from build123d import *

# Parameters (mm, degrees)
BOSS_EXTRUDE1_DEPTH = 18
SKETCH2_W           = 200
SKETCH2_H           = 118
CUT_EXTRUDE1_DEPTH  = 19
CUT_EXTRUDE2_DEPTH  = 10
SKETCH4_W           = 17.5
SKETCH4_H           = 40
SKETCH4_W_2         = 40
SKETCH4_H_2         = 17.5
SKETCH4_H_3         = 20
CUT_EXTRUDE3_DEPTH  = 19


with BuildPart() as part:
    # Sketch1 → Boss-Extrude1 (new body)
    with BuildSketch(Plane.XY):
        with BuildLine():
            Line((0, 0), (51.303021499, -140.953893118))
            Line((51.303021499, -140.953893118), (-5.078535748, -161.475101717))
            ThreePointArc((-5.078535748, -161.475101717), (-63.089907624, -263.513472234), (-48.666413819, -380))
            Line((-48.666413819, -380), (-491.60308739, -380))
            ThreePointArc((-491.60308739, -380), (-536.64849181, -170.176041514), (-749.936822659, -193.909350133))
            ThreePointArc((-749.936822659, -193.909350133), (-806.401902791, -197.329105332), (-809.82165799, -140.864025199))
            ThreePointArc((-809.82165799, -140.864025199), (-704.170284695, -71.694204299), (-578.030994047, -65.731305902))
            ThreePointArc((-578.030994047, -65.731305902), (-333.746195792, -84.570747443), (-93.969262079, -34.202014333))
            Line((-93.969262079, -34.202014333), (0, 0))
        make_face()
    extrude(amount=BOSS_EXTRUDE1_DEPTH)

    # Sketch2 → Cut-Extrude1 (cut, through all)
    with BuildSketch(Plane.XY.offset(18)):
        with Locations((-187.508312236, -271)):
            Rectangle(SKETCH2_W, SKETCH2_H)
        with BuildLine():
            Line((-322.508312236, -360), (-432.508312236, -360))
            Line((-432.508312236, -360), (-432.508312236, -300))
            ThreePointArc((-432.508312236, -300), (-377.508312236, -245), (-322.508312236, -300))
            Line((-322.508312236, -300), (-322.508312236, -360))
        make_face()
    extrude(amount=-CUT_EXTRUDE1_DEPTH, mode=Mode.SUBTRACT)

    # Sketch3 → Cut-Extrude2 (cut)
    with BuildSketch(Plane.XY.offset(18)):
        Polygon((-1.01570715, -32.295020343), (29.76610575, -116.867356214), (-4.062828599, -129.180081374), (-34.844641498, -44.607745503), align=None)
    extrude(amount=-CUT_EXTRUDE2_DEPTH, mode=Mode.SUBTRACT)

    # Sketch4 → Cut-Extrude3 (cut, through all)
    with BuildSketch(Plane.XY.offset(18)):
        with Locations((-630.167151995, -140)):
            Rectangle(SKETCH4_W, SKETCH4_H)
        with Locations((-470.167151995, -300)):
            Rectangle(SKETCH4_W_2, SKETCH4_H_2)
        with Locations((-296.258312236, -272)):
            Rectangle(SKETCH4_W, SKETCH4_H_3)
    extrude(amount=-CUT_EXTRUDE3_DEPTH, mode=Mode.SUBTRACT)


solid = part.part
Can you work these out from the model? Positions are in its coordinate system, mm. A direction names the side the tool comes from. Round coordinates to 2 decimals unless told otherwise and drop trailing zeros. Write each loop counter-clockwise with the first axis right and the second up, starting at its lowest first coordinate (ties: lowest second). Pieces come first, ordered by that corner, then holes. Notation, with made-up numbers: (71.25, 6.25) - (130.25, 6.25) arc R31 ccw to (130.25, 38.25) - close; hole circle Ø5 at (-18, 47.5). An arc over 180 degrees is marked (long way). Write each question's results on one line, items separated by ' | '. Start each with the question number.
1) Suppose I cut it at D-D (x = -128). List the corners of the cut face in (y, z) for me.
2) Suppose I cut it at A-A (x = -254.5). List the corners of the cut face in (y, z) for me.
3) Suppose I cut it at B-B (z = 5). Give the number of separate pieces and of enclosed holes in the cut face, and give its area (3 significant figures).
4) For pin 1 Ø6 at (x, z) = (-689.5, 10.5) entering from +Y; pin 2 Ø5.5 at (y, z) = (-269, 12.5) entering from +X; pin 3 Ø1 at (x, z) = (-217, 6.5) entering from +Y, each with a flat end and sliding along its axis, tell me the tip position at first contact or that it passes through.
5) We'd pull the mould along X, two halves only. Please class faces 4 (the flat face through (-350, -175, 18)), 5 (the flat face through (-287.508, -306, 9)), 6 (the flat face through (-87.508, -272, 9)), 7 (the cylindrical face through (-476.96, -346.13, 8.87)): released by +X, released by -X, zero draft, split by the parting line, or undercut.
6) Suppose I cut it at C-C (x = -710). List the corners of the cut face in (y, z) for me, and give its area (3 significant figures).
7) Please list where these lines run through material, in increasing order: line 1 (X direction, y = -280, z = 6.5); line 2 (X direction, y = -317, z = 3.75); line 3 (X direction, y = -129.5, z = 10.75).
8) Which directions (+Z, -Z, +X, -X, +Y, -Y) give clear straight access to the entire face, cutting with the end or side of a thin tool? Please do faces 1 (the flat face through (-460, -308.75, 9)), 2 (the flat face through (-296, -282, 9)), 3 (the flat face through (-19.238, -87.486, 13.07)).
Here are the results:
1) outline: (-380, 0) - (-330, 0) - (-330, 18) - (-380, 18) - close; (-212, 0) - (-45.79, 0) - (-45.79, 18) - (-212, 18) - close
2) outline: (-380, 0) - (-330, 0) - (-330, 18) - (-380, 18) - close; (-212, 0) - (-75.73, 0) - (-75.73, 18) - (-212, 18) - close
3) separate pieces: 1 | enclosed holes: 2 | area: 139,000 mm2
4) pin 1: stops at y = -66.7 | pin 2: stops at x = -63.61 | pin 3: stops at y = -68.83
5) face 4: zero draft | face 5: undercut | face 6: undercut | face 7: released by -X
6) outline: (-161.34, 0) - (-73.67, 0) - (-73.67, 18) - (-161.34, 18) - close | area: 1,580 mm2
7) line 1: x = -471.42 to -428.74, -326.27 to -305.01, -87.51 to -65.62 | line 2: x = -471.07 to -432.51, -322.51 to -287.51, -87.51 to -65.92 | line 3: x = -799.07 to -638.92, -621.42 to 47.13
8) face 1: +Z, -Z, -X | face 2: +Z, -Z | face 3: +Z
